Geometry: see drawing. Coordinates: mm, zero at the bounding-box minimum. A direction names the side the tool comes from. Coordinates: 2 decimals unless noted, no trailing zeros. Order: outer loops, then holes, each group sorted by start corner. A loop starts at its lowest first (then second) coordinate and runs counter-clockwise, first axis right, second up.
Item 1: Section B-B on y = 9. Return the cut outline in (x, z), then the cut area to 3 significant figures.
Item 2: Contact query for flat-ended pins moving along their axis: P1, Ø8, axis at x = 26.5, y = 7.5, coming from the +Z side; P2, Ø6, axis at y = 6.5, z = 14, coming from the +X side; P3, Ø1.5, axis at x = 42, z = 10, coming from the +Y side. Output: stop coordinate, or through.
Item 3: Section C-C on y = 3.75. Return the cut outline in (x, z).
Item 4: Section D-D on z = 13.25. Return the cut outline in (x, y).
Item 5: Ray query, line 1 (Y direction, x = 27, z = 3); line 2 (Z direction, x = 32, y = 11.5); line 3 (X direction, y = 11.25, z = 9). Return the intervals inside material, ascending.
Item 6: Section A-A on z = 10.75. Return the cut outline in (x, y).
Item 7: Reachability of the marked faces 1 and 2 from +Z, -Z, +X, -X, +Y, -Y: full face, straight path, thin tool, end or side. Return the list, or none.
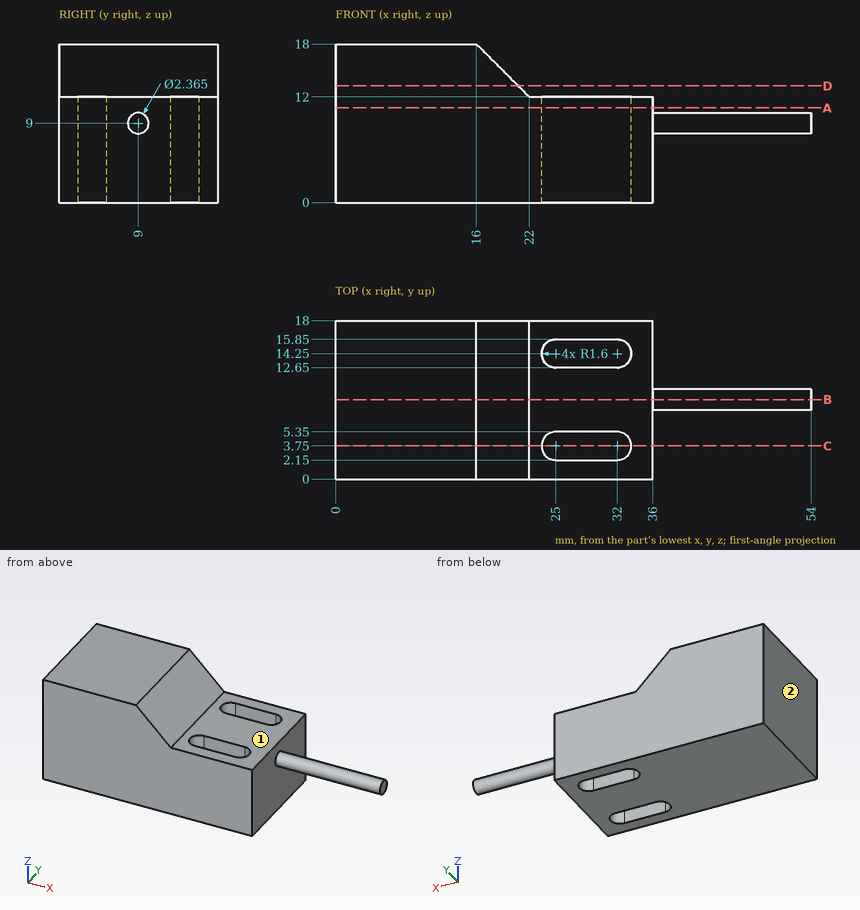
Answer list:
1. outline: (0, 0) - (36, 0) - (36, 7.82) - (54, 7.82) - (54, 10.18) - (36, 10.18) - (36, 12) - (22, 12) - (16, 18) - (0, 18) - close
1. area: 589 mm2
2. P1: stops at z = 12
2. P2: stops at x = 36
2. P3: stops at y = 10.16
3. outline: (0, 0) - (23.4, 0) - (23.4, 12) - (22, 12) - (16, 18) - (0, 18) - close; (33.6, 0) - (36, 0) - (36, 12) - (33.6, 12) - close
4. outline: (0, 0) - (20.75, 0) - (20.75, 18) - (0, 18) - close
5. line 1: y = 0 to 2.15, 5.35 to 12.65, 15.85 to 18
5. line 2: z = 0 to 12
5. line 3: x = 0 to 36
6. outline: (0, 0) - (36, 0) - (36, 18) - (0, 18) - close; hole (25, 2.15) - (32, 2.15) arc R1.6 ccw to (32, 5.35) - (25, 5.35) arc R1.6 ccw to start; hole (25, 12.65) - (32, 12.65) arc R1.6 ccw to (32, 15.85) - (25, 15.85) arc R1.6 ccw to start
7. face 1: +Z, +X, +Y, -Y
7. face 2: +Z, -Z, -X, +Y, -Y
